Autodesk Inventor part; units mm, degrees
ref_plane "YZ Plane" through (0, 0, 0) normal (1, 0, 0) x (0, 1, 0)
ref_plane "XZ Plane" through (0, 0, 0) normal (0, 1, 0) x (-1, 0, 0)
ref_plane "XY Plane" through (0, 0, 0) normal (0, 0, 1) x (1, 0, 0)
sketch "Sketch1" plane through (0, 0, 0) normal (0, 0, 1) x (1, 0, 0)
  line L0 (18.5864, 6.043) -> (94.7864, 6.043)
  line L1 (94.7864, 6.043) -> (94.7864, -44.757)
  line L2 (94.7864, -44.757) -> (18.5864, -44.757)
  line L3 (18.5864, -44.757) -> (18.5864, 6.043)
  point P0 (0, 0)
  dimension "d0" = 76.2
  dimension "d1" = 50.8
extrude "Extrusion1" add sketch "Sketch1" along normal blind 50.8
sketch "Sketch2" plane through (94.7864, -44.757, 0) normal (1, 0, 0) x (0, 0, -1)
  line L0 (0, 50.8) -> (-50.8, 50.8)
  line L1 (0, 0) -> (-50.8, 0)
  line L2 (-50.8, 50.8) -> (-25.4, 50.8)
  line L3 (-25.4, 50.8) -> (-25.4, 0)
  line L4 (-25.4, 0) -> (-50.8, 0)
  line L5 (-50.8, 0) -> (-50.8, 50.8)
  point P0 (0, 44.757)
  dimension "d4" = 25.4
extrude "Extrusion2" cut sketch "Sketch2" against normal blind 50.8
sketch "Sketch3" plane through (18.5864, -44.757, 0) normal (-1, 0, 0) x (0, 0, 1)
  point P0 (0, 44.757)
sketch "Sketch4" plane through (18.5864, -44.757, 0) normal (-1, 0, 0) x (0, 0, 1)
  line L0 (0, 0) -> (50.8, 0)
  line L1 (50.8, 0) -> (25.4, 0)
  line L2 (25.4, 0) -> (25.4, 26.8957)
  line L3 (25.4, 26.8957) -> (50.8, 26.8957)
  line L4 (50.8, 26.8957) -> (50.8, 0)
  point P0 (0, 44.757)
  dimension "d7" = 25.4
extrude "Extrusion3" cut sketch "Sketch4" against normal blind 50.8
sketch "Sketch5" plane through (94.7864, -44.757, 25.4) normal (0, 0, 1) x (1, 0, 0)
  line L0 (-50.8, 50.8) -> (0, 50.8)
  line L1 (0, 50.8) -> (-25.4, 50.8)
  line L2 (-25.4, 50.8) -> (-25.4, 25.4)
  line L3 (-25.4, 25.4) -> (0, 25.4)
  line L4 (0, 25.4) -> (0, 50.8)
  point P0 (-94.7864, 44.757)
  dimension "d10" = 25.4
  dimension "d11" = 25.4
extrude "Extrusion4" cut sketch "Sketch5" against normal blind 50.8
properties part number "Ied Final"
Check sheet for the modelled part. Datum: model origin and axes. Units: mm. A direction names the side the tool comes from. Round coordinates to 2 decimals unless told otherwise and drop trailing zeros. Loops run counter-clockwise (first coordinate to the right, second up) from the corner with the lowest first, then second, coordinate; pieces in that order, holes last. Notation, with made-up numbers: M 61.25,81.25 L 72.25,81.25 A23 ccw 72.25,101.25 Z; hole C -33.5,26 d4. An arc over 180 degrees is marked long. One line per question, with ' | ' between items. Start each with the question number.
Item 1: Section check A-A (z = 16). Record the boundary of the cut face in (x, y).
Item 2: Section check D-D (x = 79). Record the boundary of the cut face in (y, z).
Item 3: Section check C-C (x = 27.5). Record the boundary of the cut face in (y, z), and give its area (3 significant figures).
Item 4: Section check B-B (y = -31). Record the boundary of the cut face in (x, z).
Item 5: Gauge pin test, flat ends, axial feed: pin 1 Ø6 at (x, y) = (60.5, -27) entering from +Z; pin 2 Ø20.5 at (x, z) = (87.5, 12) entering from +Y; pin 3 Ø12.5 at (x, z) = (28.5, 40.5) entering from -Y. Record the tip position at first contact, or that the pin passes through.
Item 6: Scan lines: probe 1 along X at (y, z) = (3.5, 21); probe 2 along Z at (x, y) = (64, -28); probe 3 along X at (y, z) = (-8, 41.5). Record each from-to range of solid material in increasing order.
Item 7: Set-up check for faces 1 (the face through (43.986, -6, 38)), 2 (the face through (31, -17.861, 38)), 3 (the face through (82, -19.357, 13)): record each of +Z, -Z, +X, -X, +Y, -Y from which the full face is reachable in a straight line by a thin tool's end or side.
Worked out:
1) outline: M 18.59,-44.76 L 94.79,-44.76 L 94.79,-19.36 L 69.39,-19.36 L 69.39,6.04 L 18.59,6.04 Z
2) outline: M -44.76,0 L -19.36,0 L -19.36,25.4 L -44.76,25.4 Z
3) outline: M -44.76,0 L 6.04,0 L 6.04,50.8 L -17.86,50.8 L -17.86,25.4 L -44.76,25.4 Z | area: 1,900 mm^2
4) outline: M 18.59,0 L 94.79,0 L 94.79,25.4 L 18.59,25.4 Z
5) pin 1: z = 25.4 | pin 2: y = -19.36 | pin 3: y = -17.86
6) probe 1: 18.59 to 69.39 | probe 2: 0 to 25.4 | probe 3: 18.59 to 43.99
7) face 1: +Z, +X, +Y, -Y | face 2: +Z, +X, -X, -Y | face 3: +Z, -Z, +X, +Y
